The drawing under review shows one solid part. Ordinate dimensions are in mm from its lowest x, y, z. A direction names the side the tool comes from. Give positions to 0.01 mm unless a question says otherwise; leave off trailing zeros. Order: outer loops, then holes, each group sorted by start corner. A loop starts at its lowest first (then second) coordinate and runs counter-clockwise, first axis right, second up. Notation, with made-up numbers: (35, -18.75) - (69, -18.75) arc R32 ccw to (69, 13.25) - close; hole circle Ø8 at (-13, 57.5). An arc over 180 degrees is marked (long way). Use CSV: the item, a comma, the result in double quotes.
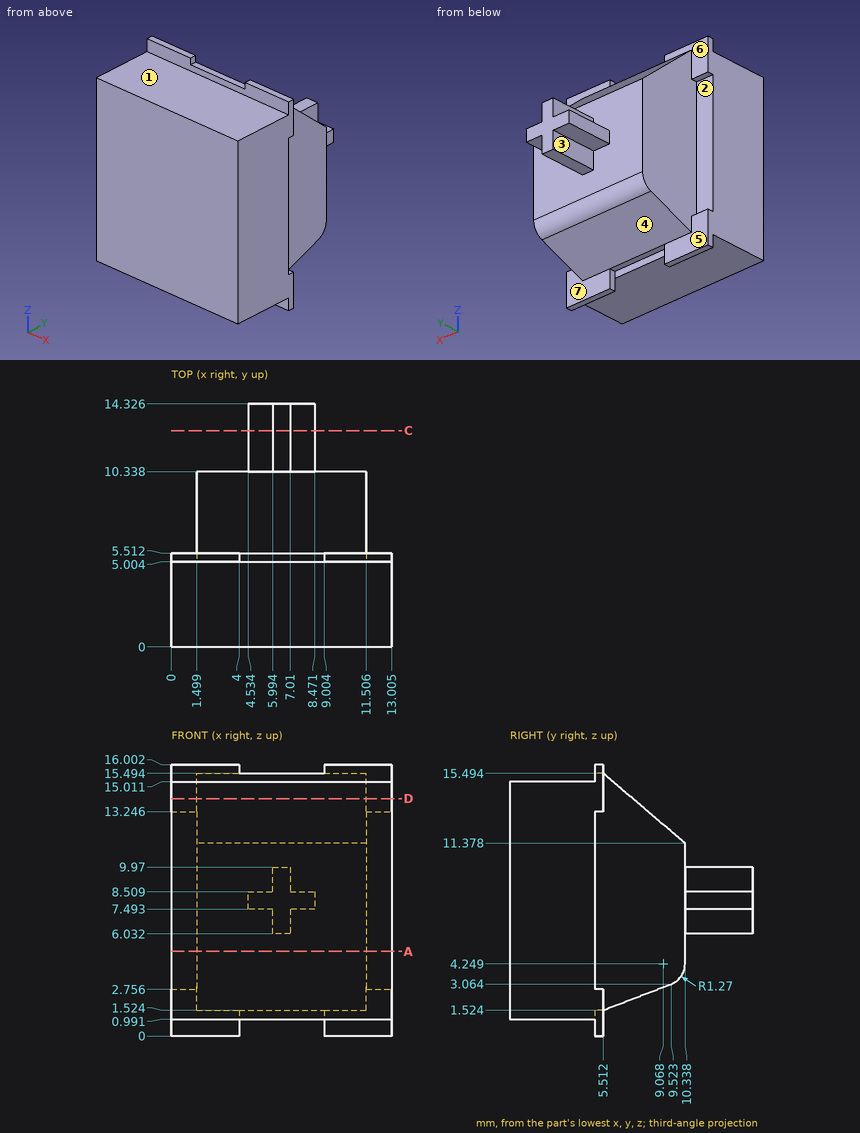
Item 1: Wall thickness on L1, parallel to Y at x = 11.75, z = 9.25; L2, parallel to Y at x = 7.5, z = 6.5; L3, parallel to Z at x = 1.75, y = 4.25: over which ranges is each line inside the solid? List them lowest first.
Results list:
L1,"y = 0 to 5"
L2,"y = 0 to 10.34"
L3,"z = 0.99 to 15.01"
Item 2: Take a section at A-A, the plane z = 5. Give the boundary of the cut face in (x, y) (1 decimal).
Results list:
outline,"(0, 0) - (13, 0) - (13, 5) - (11.5, 5) - (11.5, 10.3) - (1.5, 10.3) - (1.5, 5) - (0, 5) - close"
Item 3: Tool access review of the marked faces 5, 6 and 7: name each direction out of +Z, -Z, +X, -X, +Y, -Y from which nothing blocks a thin tool from reaching the whole face with its end or side.
Results list:
face 5,"-Z, -X, +Y"
face 6,"+Z, -X, +Y"
face 7,"-Z, +X, +Y"
Item 4: Mouldability with a two-part tool opening along Z and no side actions: class the marked faces 1, 2, 3 and 4 as pulls with the +Z half, pulls with the -Z half, needs draft (parallel to the pull), parting line crosses it, or undercut.
Results list:
face 1,"pulls with the +Z half"
face 2,"undercut"
face 3,"needs draft"
face 4,"pulls with the -Z half"
Item 5: Clearance check with flat-ended pins moving along their axes: pin 1 (2 mm diameter, centred on y = 11.5, z = 10.5, fed in from -X); pin 2 (1.6 mm diameter, centred on x = 0.5, z = 5.5, fed in from +Y); pin 3 (1.6 mm diameter, centred on y = 8.5, z = 8, fed in from -X). State where each tip first meets the part, or that it passes through.
Results list:
pin 1,"stops at x = 5.99"
pin 2,"stops at y = 5"
pin 3,"stops at x = 1.5"
Item 6: Take a section at C-C, the plane y = 12.75. Give the boundary of the cut face in (x, z) (1 decimal).
Results list:
outline,"(4.5, 7.5) - (6, 7.5) - (6, 6) - (7, 6) - (7, 7.5) - (8.5, 7.5) - (8.5, 8.5) - (7, 8.5) - (7, 10) - (6, 10) - (6, 8.5) - (4.5, 8.5) - close"
Item 7: Take a section at D-D, the plane z = 14. Give the boundary of the cut face in (x, y) (1 decimal), and give its area (3 significant figures).
Results list:
outline,"(0, 0) - (13, 0) - (13, 5.5) - (11.5, 5.5) - (11.5, 7.3) - (1.5, 7.3) - (1.5, 5.5) - (0, 5.5) - close"
area,"89.2 mm2"
